For this review, take the finished solid that the model builds, in its own axes (mm). Coordinates: 2 decimals unless noted, no trailing zeros. Write each loop counter-clockwise with the first axis right and the second up, starting at its lowest first coordinate (ties: lowest second). Pieces come first, ordered by that corner, then holes. Notation, with made-up numbers: (-28, 22.25) -> (26, 22.25) arc R11 ccw to (26, 33.25) -> close; hole circle Ø1 at (75.5, 81.25). An arc over 180 degrees is marked (long way). Put each result on its own line as item: value. Start each with the question number.
Item 1: To check wall thickness, follow L1, parallel to X at y = -8, z = 157; L2, parallel to Z at x = 4, y = -0.5; L3, parallel to Y at x = 7, z = 466.5. State the ranges of each line that lie inside material, in increasing order.
Item 2: Consider section A-A on z = 619. Give the boundary of the cut face in (x, y).
Item 3: Insertion check: P1, Ø7.5, axis at y = -8.92, z = 383.54, coming from the +X side; P2, Ø5, axis at y = -8.92, z = 251.46, coming from the -X side. Each pin has a flat end and moves straight along its axis. Give the tip position at first contact, or say it passes through.
Item 4: Consider section B-B on z = 184. Give the boundary of the cut face in (x, y).
Item 5: Consider section C-C on z = 342.9. Give the boundary of the cut face in (x, y).
```python
from build123d import *

# Parameters (mm, degrees)
SKETCH1_W                    = 31.75
SKETCH1_H                    = 63.5
SKETCH1_W_2                  = 25.4
SKETCH1_H_2                  = 57.15
BOSS_EXTRUDE1_DEPTH          = 685.8
CUT_EXTRUDE1_REACH           = 691.238
F_10_0_1935_DIAMETER_HOLE1_D = 4.9149
CUT_EXTRUDE2_START           = -31.75
SKETCH6_R                    = 14.2875
SKETCH6_R_2                  = 3.2639
SKETCH6_R_3                  = 2.413
CUT_EXTRUDE2_DEPTH           = 31.75


with BuildPart() as part:
    # Sketch1 → Boss-Extrude1 (new body)
    with BuildSketch(Plane.XY):
        with Locations((3.710272719, -29.23968021)):
            Rectangle(SKETCH1_W, SKETCH1_H)
        with Locations((3.710272719, -29.23968021)):
            Rectangle(SKETCH1_W_2, SKETCH1_H_2, mode=Mode.SUBTRACT)
    extrude(amount=BOSS_EXTRUDE1_DEPTH)

    # Cut-Extrude1: up to this face of the body (flat: up to its plane)
    cut_extrude1_end = Plane(part.part.faces().sort_by_distance((19.585272719, -29.23968021, 342.9))[0])
    # Sketch3 → Cut-Extrude1 (cut, up to the picked face)
    with BuildSketch(Plane.ZY.offset(12.164727281), mode=Mode.PRIVATE) as cut_extrude1_sk1:
        with BuildLine():
            Line((31.7754, -13.36468021), (120.6754, -13.36468021))
            ThreePointArc((120.6754, -13.36468021), (122.92046403, -14.294616179), (123.8504, -16.53968021))
            Line((123.8504, -16.53968021), (123.8504, -41.93968021))
            ThreePointArc((123.8504, -41.93968021), (122.92046403, -44.18474424), (120.6754, -45.11468021))
            Line((120.6754, -45.11468021), (31.7754, -45.11468021))
            ThreePointArc((31.7754, -45.11468021), (29.53033597, -44.18474424), (28.6004, -41.93968021))
            Line((28.6004, -41.93968021), (28.6004, -16.53968021))
            ThreePointArc((28.6004, -16.53968021), (29.53033597, -14.294616179), (31.7754, -13.36468021))
        make_face()
    cut_extrude1_tool1 = split(extrude(cut_extrude1_sk1.sketch, amount=-CUT_EXTRUDE1_REACH, mode=Mode.PRIVATE), bisect_by=cut_extrude1_end, keep=Keep.BOTH, mode=Mode.PRIVATE)
    # Sketch3 → Cut-Extrude1 (cut, up to the picked face)
    with BuildSketch(Plane.ZY.offset(12.164727281), mode=Mode.PRIVATE) as cut_extrude1_sk2:
        with BuildLine():
            ThreePointArc((657.1996, -41.93968021), (656.26966403, -44.18474424), (654.0246, -45.11468021))
            Line((654.0246, -45.11468021), (565.1246, -45.11468021))
            ThreePointArc((565.1246, -45.11468021), (562.87953597, -44.18474424), (561.9496, -41.93968021))
            Line((561.9496, -41.93968021), (561.9496, -16.53968021))
            ThreePointArc((561.9496, -16.53968021), (562.87953597, -14.294616179), (565.1246, -13.36468021))
            Line((565.1246, -13.36468021), (654.0246, -13.36468021))
            ThreePointArc((654.0246, -13.36468021), (656.26966403, -14.294616179), (657.1996, -16.53968021))
            Line((657.1996, -16.53968021), (657.1996, -41.93968021))
        make_face()
    cut_extrude1_tool2 = split(extrude(cut_extrude1_sk2.sketch, amount=-CUT_EXTRUDE1_REACH, mode=Mode.PRIVATE), bisect_by=cut_extrude1_end, keep=Keep.BOTH, mode=Mode.PRIVATE)
    add(cut_extrude1_tool1.solids().sort_by(Axis((-12.164727, -29.23968, 76.2254), (1, 0, 0)))[0], mode=Mode.SUBTRACT)
    add(cut_extrude1_tool2.solids().sort_by(Axis((-12.164727, -29.23968, 609.5746), (1, 0, 0)))[0], mode=Mode.SUBTRACT)

    # #10 (0.1935) Diameter Hole1 (through all)
    with Locations(Plane(origin=(3.710272719, 2.51031979, 677.8625), x_dir=(1, 0, 0), z_dir=(0, 1, 0))):
        with Locations((0, 0), (0, 669.925)):
            Hole(F_10_0_1935_DIAMETER_HOLE1_D / 2)

    # Sketch6 → Cut-Extrude2 (cut)
    with BuildSketch(Plane(origin=(19.585272719, 0, 0), x_dir=(0, 0, -1), z_dir=(1, 0, 0)).offset(CUT_EXTRUDE2_START)):
        with Locations(Location((-342.9, -34.00218021, 0), (0, 0, 90))):
            Circle(SKETCH6_R)
        with Locations(Location((-383.54, -8.91968021, 0), (0, 0, 90))):
            Circle(SKETCH6_R_2)
        with Locations(Location((-251.46, -8.91968021, 0), (0, 0, 90))):
            Circle(SKETCH6_R_2)
        with Locations(Location((-317.5, -55.40168021, 0), (0, 0, 90))):
            Circle(SKETCH6_R_3)
        with Locations(Location((-292.1, -34.00218021, 0), (0, 0, 90))):
            Circle(SKETCH6_R)
    extrude(amount=CUT_EXTRUDE2_DEPTH, mode=Mode.SUBTRACT)


solid = part.part
```
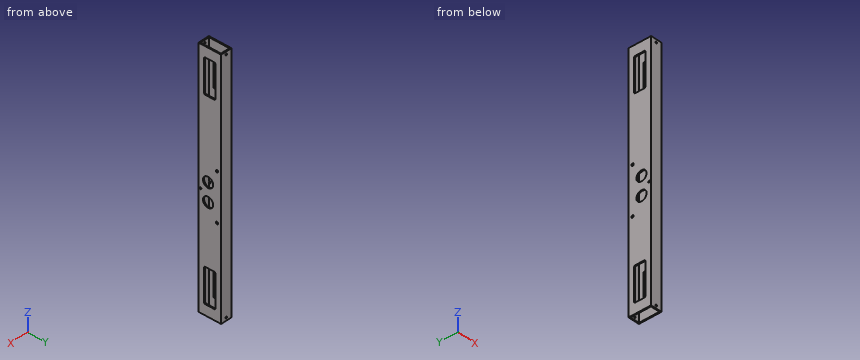
Return value:
1. L1: -12.16 to -8.99, 16.41 to 19.59
1. L2: 0 to 5.5, 10.38 to 675.42, 680.3 to 685.8
1. L3: -60.99 to -57.81, -0.66 to 2.51
2. outline: (-12.16, -60.99) -> (19.59, -60.99) -> (19.59, -45.11) -> (16.41, -45.11) -> (16.41, -57.81) -> (-8.99, -57.81) -> (-8.99, -45.11) -> (-12.16, -45.11) -> close; (-12.16, -13.36) -> (-8.99, -13.36) -> (-8.99, -0.66) -> (16.41, -0.66) -> (16.41, -13.36) -> (19.59, -13.36) -> (19.59, 2.51) -> (-12.16, 2.51) -> close
3. P1: x = 19.59
3. P2: through
4. outline: (-12.16, -60.99) -> (19.59, -60.99) -> (19.59, 2.51) -> (-12.16, 2.51) -> close; hole (-8.99, -57.81) -> (16.41, -57.81) -> (16.41, -0.66) -> (-8.99, -0.66) -> close
5. outline: (-12.16, -60.99) -> (19.59, -60.99) -> (19.59, -48.29) -> (16.41, -48.29) -> (16.41, -57.81) -> (-8.99, -57.81) -> (-8.99, -48.29) -> (-12.16, -48.29) -> close; (-12.16, -19.71) -> (-8.99, -19.71) -> (-8.99, -0.66) -> (16.41, -0.66) -> (16.41, -19.71) -> (19.59, -19.71) -> (19.59, 2.51) -> (-12.16, 2.51) -> close
